Autodesk Inventor part; units mm, degrees
ref_plane "YZ Plane" through (0, 0, 0) normal (1, 0, 0) x (0, 1, 0)
ref_plane "XZ Plane" through (0, 0, 0) normal (0, 1, 0) x (-1, 0, 0)
ref_plane "XY Plane" through (0, 0, 0) normal (0, 0, 1) x (1, 0, 0)
sketch "Sketch1" plane through (0, 0, 0) normal (0, 0, 1) x (1, 0, 0)
  line L0 (0, 0) -> (132, 0)
  line L1 (42.329, 220) -> (32.329, 218.2367)
  line L2 (32.329, 218.2367) -> (0, 0)
  line L3 (129, 22) -> (84, 5.6213)
  line L4 (84, 5.6213) -> (114.3391, 5.6213) construction
  line L5 (84, 5.6213) -> (42.329, 220)
  line L6 (132, 0) -> (129, 22)
  line L7 (129, 22) -> (164, 22)
  line L8 (164, 22) -> (164, 0)
  line L9 (164, 0) -> (132, 0)
  dimension "d0" = 132
  dimension "d1" = 220
  dimension "d6" = 20
  dimension "d7" = 81
  dimension "d8" = 10
  dimension "d9" = 10
  dimension "d22" = 45
  dimension "d23" = 22
  dimension "d24" = 3
extrude "Extrusion1" add sketch "Sketch1" along normal blind 1050
sketch "Sketch2" plane through (32.329, 218.2367, 1050) normal (-0.1736482, 0.9848078, 0) x (0.9848078, 0.1736482, 0)
  line L0 (0, 277) -> (10.1543, 277)
  line L1 (10.1543, 277) -> (10.1543, 247)
  line L2 (10.1543, 247) -> (0, 247)
  line L3 (0, 247) -> (0, 277)
  line L4 (0, 1050) -> (0, 0) construction
  line L5 (0, 803) -> (10.1543, 803)
  line L6 (10.1543, 803) -> (10.1543, 773)
  line L7 (10.1543, 773) -> (0, 773)
  line L8 (0, 773) -> (0, 803)
  line L9 (13.9657, 1050) -> (0, 1050) construction
  line L10 (10.1543, 1050) -> (10.1543, 0) construction
  point P0 (-69.7343, 1050)
  dimension "d12" = 30
  dimension "d13" = 30
  dimension "d14" = 247
  dimension "d15" = 247
extrude "Extrusion2" add sketch "Sketch2" along normal blind 220
fillet "Fillet1" radius 3 4 edges at (4.1264, 436.6577, 788) (-5.8736, 434.8944, 788) (4.1264, 436.6577, 262) (-5.8736, 434.8944, 262)
fillet "Fillet2" radius 10 4 edges at (37.329, 219.1184, 803) (37.329, 219.1184, 277) (37.329, 219.1184, 773) (37.329, 219.1184, 247)
properties part number "sostenedor1"
The listing builds one solid part. Answer for the finished solid, in the listing's coordinates (mm). A direction names the side the tool comes from. Give positions to 0.01 mm unless a question says otherwise; leave off trailing zeros. Write each loop counter-clockwise with the first axis right and the second up, starting at its lowest first coordinate (ties: lowest second). Pieces come first, ordered by that corner, then holes.
Item 1: Section B-B, the plane y = 269 is taken. Write down the section's boundary in (x, z).
Item 2: Which of the six approach directions +Z, -Z, +X, -X, +Y, -Y give full straight-line access (tool end or side, diameter ignored) to faces 4 (the flat face through (106.815, 13.925, 517.65)), 5 (the flat face through (146, 22, 518)), 6 (the flat face through (13.752, 323.592, 788.35))?
Item 3: Find the intervals of material crossed by line 1 along Z through (x, y) = (20, 341.5); line 2 along Y through (x, z) = (130.5, 870); line 3 along X through (y, z) = (70.5, 265), in increasing order.
Item 4: Section C-C, the plane x = 63.5 is taken. Write down the section's boundary in (y, z), plus the area to 3 significant figures.
Item 5: Section A-A, the plane z = 632 is taken. Write down the section's boundary in (x, y), plus the area to 3 significant figures.
Item 6: Determine the mould class of faces 1 (the flat face through (18, 331, 773)), 2 (the flat face through (45, 70, 0)), 3 (the flat face through (164, 11, 518)) for opening direction Z: released by +Z, released by -Z, zero draft, split by the parting line, or undercut.
Item 7: Flat-ended cylindrical pins translate along their axes: P1, Ø4, axis at y = 116.5, z = 570, coming from the -X side; P2, Ø23, axis at x = 29, y = 352, coming from the +Z side; P3, Ø2, axis at y = 45.5, z = 532.5, coming from the -X side. Find the tip coordinate at first contact, or state that the pin passes through.
Item 8: Section D-D, the plane y = 74 is taken. Write down the section's boundary in (x, z), plus the area to 3 significant figures.
Completed:
1. outline: (23.38, 247) - (33.69, 247) - (33.69, 277) - (23.38, 277) - close; (23.38, 773) - (33.69, 773) - (33.69, 803) - (23.38, 803) - close
2. face 4: +Z, -Z, +Y
2. face 5: +Z, -Z, +X, +Y
2. face 6: +Z, -Z, -X
3. line 1: z = 247 to 277, 773 to 803
3. line 2: y = 0 to 22
3. line 3: x = 10.44 to 71.39
4. outline: (0, 0) - (111.08, 0) - (111.08, 1050) - (0, 1050) - close
4. area: 117,000 mm2
5. outline: (0, 0) - (164, 0) - (164, 22) - (129, 22) - (84, 5.62) - (42.33, 220) - (32.33, 218.24) - close
5. area: 11,800 mm2
6. face 1: undercut
6. face 2: released by -Z
6. face 3: zero draft
7. P1: stops at x = 16.96
7. P2: stops at z = 803
7. P3: stops at x = 6.59
8. outline: (10.96, 0) - (70.71, 0) - (70.71, 1050) - (10.96, 1050) - close
8. area: 62,700 mm2
